Read the model definition and answer for the solid it produces. Units are mm, in the model's axes. Face numbers are marked on the shaded views. A direction names the side the tool comes from. Give positions to 0.01 mm unless a question says otherwise; leave off trailing zeros. Order: outer loops, then holes, each group sorted by start corner. A loop starts at its lowest first (then second) coordinate and runs counter-clockwise, first axis right, second up. Notation, with made-up numbers: (67.5, -1.5) -> (81.5, -1.5) arc R23 ccw to (81.5, 24.5) -> close; hole circle Ø3 at (14.5, 4.5). An arc over 180 degrees is marked (long way). One line per item, written item: value. Start each with the question number.
from build123d import *

# Parameters (mm, degrees)
F0_W      = 500
F0_H      = 500
F1_DEPTH  = 6
F3_DEPTH  = 200.09
F5_DEPTH  = 25
F8_DEPTH  = 25
F9_DEPTH  = 25
F2_R      = 15
F10_DEPTH = 25
F12_DEPTH = 25
F2_R_2    = 45
F13_DEPTH = 375


with BuildPart() as f1:
    # F0 (on Top) → F1 (new body)
    with BuildSketch(Plane.XY):
        Rectangle(F0_W, F0_H)
    extrude(amount=F1_DEPTH)

    # F2 (on face) → F3 (join)
    with BuildSketch(Plane.XY.offset(6)):
        with BuildLine():
            ThreePointArc((-3, 50.9116882454), (0, 51), (3, 50.9116882454))
            Line((3, 50.9116882454), (3, 250))
            Line((3, 250), (-3, 250))
            Line((-3, 250), (-3, 50.9116882454))
        make_face()
        with BuildLine():
            ThreePointArc((50.9116882454, 3), (50.9779172805, 1.5006497731), (51, 0))
            ThreePointArc((51, 0), (50.9779172805, -1.5006497731), (50.9116882454, -3))
            Line((50.9116882454, -3), (250, -3))
            Line((250, -3), (250, 3))
            Line((250, 3), (50.9116882454, 3))
        make_face()
        with BuildLine():
            ThreePointArc((-50.9116881716, -3.0000012524), (-51, -1.2546e-06), (-50.9116883192, 2.9999987476))
            Line((-50.9116883192, 2.9999987476), (-250, 3))
            Line((-250, 3), (-250, -3))
            Line((-250, -3), (-50.9116881716, -3.0000012524))
        make_face()
        with BuildLine():
            Line((3, -250), (3, -50.9116882454))
            ThreePointArc((3, -50.9116882454), (0, -51), (-3, -50.9116882454))
            Line((-3, -50.9116882454), (-3, -250))
            Line((-3, -250), (3, -250))
        make_face()
    extrude(amount=F3_DEPTH)

    # F4 (on face) → F5 (cut)
    with BuildSketch(Plane(origin=(0, 3, 0), x_dir=(-1, 0, 0), z_dir=(0, 1, 0))):
        Polygon((-250, 206.09), (-250, 6), (-50.9116882454, 205.0883117546), (-50.9116882454, 206.09), align=None)
    extrude(amount=-F5_DEPTH, mode=Mode.SUBTRACT)

    # F6 (on face) → F8 (cut)
    with BuildSketch(Plane.YZ.offset(3)):
        Polygon((-250, 206.09), (-250, 6), (-50.9116882454, 205.0883117546), (-50.9116882454, 206.09), align=None)
    extrude(amount=-F8_DEPTH, mode=Mode.SUBTRACT)

    # F7 (on face) → F9 (cut)
    with BuildSketch(Plane(origin=(-3, 0, 0), x_dir=(0, -1, 0), z_dir=(-1, 0, 0))):
        Polygon((-250, 206.09), (-250, 6), (-50.9116882454, 205.0883117546), (-50.9116882454, 206.09), align=None)
    extrude(amount=-F9_DEPTH, mode=Mode.SUBTRACT)

    # F2 (on face) → F10 (cut)
    with BuildSketch(Plane.XY.offset(6)):
        with Locations((-200, -200)):
            Circle(F2_R)
        with Locations((200, -200)):
            Circle(F2_R)
        with Locations((200, 200)):
            Circle(F2_R)
        with Locations((-200, 200)):
            Circle(F2_R)
    extrude(amount=-F10_DEPTH, mode=Mode.SUBTRACT)

    # F11 (on face) → F12 (cut)
    with BuildSketch(Plane(origin=(-1.89e-08, -3.0000015726, 0), x_dir=(1, -6.3e-09, 0), z_dir=(-6.3e-09, -1, 0))):
        Polygon((-249.9999999811, 206.09), (-249.9999999811, 6), (-50.9116881528, 205.0883118284), (-50.9116881528, 206.09), align=None)
    extrude(amount=-F12_DEPTH, mode=Mode.SUBTRACT)

    # F2 (on face) → F13 (join)
    with BuildSketch(Plane.XY.offset(6)):
        with BuildLine():
            ThreePointArc((50.9116882454, -3), (50.9779172805, -1.5006497731), (51, 0))
            ThreePointArc((51, 0), (50.9779172805, 1.5006497731), (50.9116882454, 3))
            ThreePointArc((50.9116882454, 3), (36.0624458405, 36.0624458405), (3, 50.9116882454))
            ThreePointArc((3, 50.9116882454), (0, 51), (-3, 50.9116882454))
            ThreePointArc((-3, 50.9116882454), (-36.0624462841, 36.062445397), (-50.9116883192, 2.9999987476))
            ThreePointArc((-50.9116883192, 2.9999987476), (-51, -1.2546e-06), (-50.9116881716, -3.0000012524))
            ThreePointArc((-50.9116881716, -3.0000012524), (-36.062445397, -36.0624462841), (-3, -50.9116882454))
            ThreePointArc((-3, -50.9116882454), (0, -51), (3, -50.9116882454))
            ThreePointArc((3, -50.9116882454), (36.0624458405, -36.0624458405), (50.9116882454, -3))
        make_face()
        Circle(F2_R_2, mode=Mode.SUBTRACT)
    extrude(amount=F13_DEPTH)


solid = f1.part
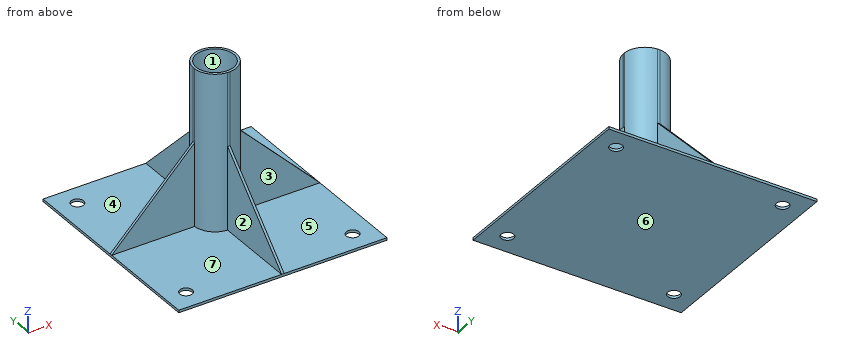
Item 1: Find section B-B on z = 176.5. Write down the section's boundary in (x, y), then the cut area to 3 significant figures.
Item 2: Find section A-A on x = 200. Write down the section's boundary in (y, z).
Item 3: Flat-ended cylindrical pins translate along their axes: pin 1 (1 mm diameter, centred on y = -116.5, z = 127, fed in from -X); pin 2 (10 mm diameter, centred on x = -39, y = -67, fed in from +Z); pin 3 (6 mm diameter, centred on y = 39, z = 74, fed in from +X). Find the tip coordinate at first contact, or state that the pin passes through.
Item 4: A tool of negligible diameter and unlimited length cuts with its end or side. For the marked faces 4, 5, 6 and 7, from which of +Z, -Z, +X, -X, +Y, -Y can it reach the whole face along a straight path? Write none if from no direction.
Item 5: Find the intervals of material crossed by line 1 (Y direction, x = -200, z = 2); line 2 (Z direction, x = -110, y = -131.5); line 3 (X direction, y = -0.5, z = 70.5), in increasing order. Write a range as from..to.
Item 6: For a pull along X with two mould halves and no side action, classify the marked faces 1, 2 and 3 as +X half, -X half, draft (parallel to the pull), parting line (faces both ways), or undercut.
Item 7: Find section D-D on y = -142.5. Write down the section's boundary in (x, z), then the cut area to 4 significant figures.
Checks:
1. outline: (-79.5, -3) -> (-50.91, -3) arc R51 ccw to (-3, -50.91) -> (-3, -79.5) -> (3, -79.5) -> (3, -50.91) arc R51 ccw to (50.91, -3) -> (79.5, -3) -> (79.5, 3) -> (50.91, 3) arc R51 ccw to (3, 50.91) -> (3, 79.5) -> (-3, 79.5) -> (-3, 50.91) arc R51 ccw to (-50.91, 3) -> (-79.5, 3) -> close; hole circle Ø90 at (0, 0)
1. area: 2,490 mm2
2. outline: (-250, 0) -> (-215, 0) -> (-215, 6) -> (-250, 6) -> close; (-185, 0) -> (185, 0) -> (185, 6) -> (3, 6) -> (3, 56) -> (-3, 56) -> (-3, 6) -> (-185, 6) -> close; (215, 0) -> (250, 0) -> (250, 6) -> (215, 6) -> close
3. pin 1: x = -3
3. pin 2: z = 6
3. pin 3: x = 36.12
4. face 4: +Z, -X, +Y
4. face 5: +Z, +X, -Y
4. face 6: -Z, +X, -X, +Y, -Y
4. face 7: +Z, -X, -Y
5. line 1: -250..-215, -185..185, 215..250
5. line 2: 0..6
5. line 3: -185.5..-45, 45..185.5
6. face 1: undercut
6. face 2: -X half
6. face 3: draft
7. outline: (-250, 0) -> (250, 0) -> (250, 6) -> (3, 6) -> (3, 113.5) -> (-3, 113.5) -> (-3, 6) -> (-250, 6) -> close
7. area: 3,645 mm2
